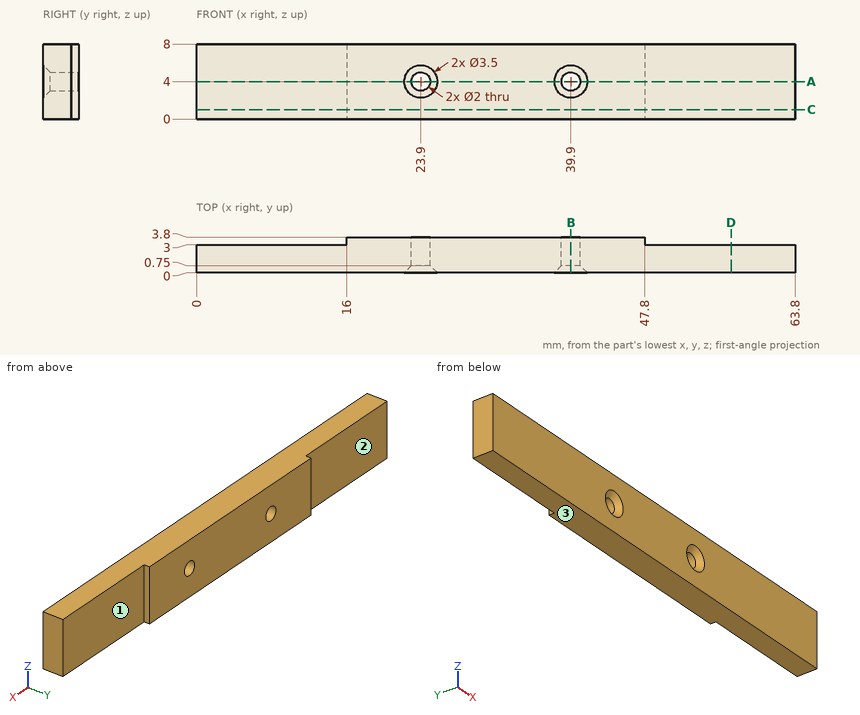
The figure shows three views and two pictorial views of one solid part (mm, origin at its lowest corner). Answer the questions. A direction names the side the tool comes from. Give positions to 0.01 mm unless a question says otherwise; leave off trailing zeros. Write each loop counter-clockwise with the first axis right and the second up, starting at its lowest first coordinate (ties: lowest second). Pieces come first, ordered by that corner, then holes. Notation, with made-up numbers: M 47.5,77.25 L 75.5,77.25 A18 ccw 75.5,95.25 Z; hole C 20.25,34 d6. An arc over 180 degrees is marked long. One line per item, written item: value. Start each with the question number.
(1) A tool of negligible diameter and unlimited length cuts with its end or side. For the marked faces 1, 2 and 3, from which of +Z, -Z, +X, -X, +Y, -Y can it reach the whole face along a straight path? Write none if from no direction.
(2) Flat-ended cylindrical pins translate along their axes: pin 1 Ø3 at (x, z) = (39.9, 4) entering from -Y; pin 2 Ø0.9 at (y, z) = (3.5, 2.5) entering from -X; pin 3 Ø2.5 at (x, z) = (23.9, 4) entering from -Y. Find the tip coordinate at first contact, or state that the pin passes through.
(3) Find section A-A (z = 4). Determine the outline of the cut face in (x, y), plus the area to 3 significant figures.
(4) Find section B-B (x = 39.9). Determine the outline of the cut face in (y, z).
(5) Find section D-D (x = 57). Determine the outline of the cut face in (y, z), plus the area to 3 significant figures.
(6) Find the intervals of material crossed by line 1 (X direction, y = 2.05, z = 4); line 2 (X direction, y = 3.05, z = 4); line 3 (Z direction, x = 39.9, y = 1.9), in increasing order.
(7) Find section C-C (z = 1). Determine the outline of the cut face in (x, y), plus the area to 3 significant figures.
Results below:
1. face 1: +Z, -Z, +X, +Y
1. face 2: +Z, -Z, -X, +Y
1. face 3: -Z, +X, -X, +Y, -Y
2. pin 1: stops at y = 0.25
2. pin 2: stops at x = 16
2. pin 3: stops at y = 0.5
3. outline: M 0,0 L 22.15,0 L 22.9,0.75 L 22.9,3.8 L 16,3.8 L 16,3 L 0,3 Z; M 24.9,0.75 L 25.65,0 L 38.15,0 L 38.9,0.75 L 38.9,3.8 L 24.9,3.8 Z; M 40.9,0.75 L 41.65,0 L 63.8,0 L 63.8,3 L 47.8,3 L 47.8,3.8 L 40.9,3.8 Z
3. area: 201 mm^2
4. outline: M 0,0 L 3.8,0 L 3.8,3 L 0.75,3 L 0,2.25 Z; M 0,5.75 L 0.75,5 L 3.8,5 L 3.8,8 L 0,8 Z
5. outline: M 0,0 L 3,0 L 3,8 L 0,8 Z
5. area: 24.0 mm^2
6. line 1: x = 0 to 22.9, 24.9 to 38.9, 40.9 to 63.8
6. line 2: x = 16 to 22.9, 24.9 to 38.9, 40.9 to 47.8
6. line 3: z = 0 to 3, 5 to 8
7. outline: M 0,0 L 63.8,0 L 63.8,3 L 47.8,3 L 47.8,3.8 L 16,3.8 L 16,3 L 0,3 Z
7. area: 217 mm^2
